Model file for the job. Use its own axes, mm. Face numbers are marked on the shaded views. Give positions to 0.01 mm unless a question says otherwise; leave off trailing zeros. Write each loop counter-clockwise with the first axis right and the second up, starting at its lowest first coordinate (ties: lowest second). Pieces come first, ordered by that corner, then holes. Notation, with made-up numbers: M 73,76.5 L 107,76.5 A24 cw 107,109.5 Z; hole C 81,-18 d9. An arc over 180 degrees is marked long. Answer as a JSON object with one key per item and string values. Group by question number.
```python
from build123d import *

# Parameters (mm, degrees)
CYLINDER002_R     = 1.5
CYLINDER002_DEPTH = 20
BOX033_W          = 12
BOX033_H          = 10
BOX033_DEPTH      = 12
FILLET011_R       = 4.5
FILLET012_R       = 4.6


with BuildPart() as cylinder:
    # Cylinder002 → Cylinder002 (new body)
    with BuildSketch(Plane(origin=(-103.2, 5, -48.3), x_dir=(1, 0, 0), z_dir=(0, 0, 1))):
        Circle(CYLINDER002_R)
    extrude(amount=CYLINDER002_DEPTH)


with BuildPart() as fillet012:
    # Box033 → Box033 (new body)
    with BuildSketch(Plane(origin=(-108.3, 0, -49.2), x_dir=(1, 0, 0), z_dir=(0, 0, 1))):
        with Locations((6, 5)):
            Rectangle(BOX033_W, BOX033_H)
    extrude(amount=BOX033_DEPTH)

    # Cut017: cut Cylinder
    add(cylinder.part, mode=Mode.SUBTRACT)

    # Fillet011
    fillet011_edges = [fillet012.edges().sort_by_distance(p)[0] for p in [
        (-108.3, 10, -43.2),
    ]]
    fillet(fillet011_edges, radius=FILLET011_R)

    # Fillet012
    fillet012_edges = [fillet012.edges().sort_by_distance(p)[0] for p in [
        (-108.3, 0, -43.2),
    ]]
    fillet(fillet012_edges, radius=FILLET012_R)


with BuildPart() as fillet012_1:
    # Fillet012 placement: moved
    add(fillet012.part.moved(Location((40.69, -41.14, 42.87))))


solid = fillet012_1.part
```
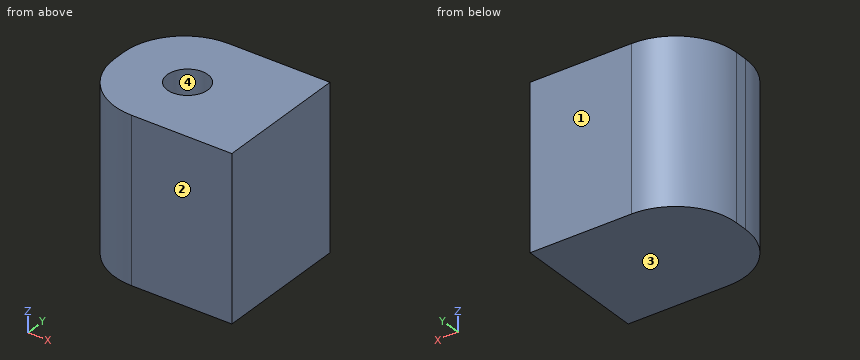
Q1. Two-plate mould, pull along Y, no slides. Class the marked faces 1, 2, 3 and 4: +Y half, -Y half, draft (parallel to the pull), parting line (faces both ways), or undercut.
Q2. Wall check: L1, parallel to X at y = -36.14, z = 2; L2, parallel to X at y = -36.5, z = -4.75; L3, parallel to X at y = -38, z = -1.25. Give the ranges that are in metal, low to high.
Q3. Drop flat-ended pins along their axis: P1, Ø2, axis at y = -33.5, z = 3, coming from the -X side; P2, Ø1, axis at x = -65, z = 1, coming from the +Y side. Give the stop position or say it passes through.
Q4. Slice it at B-B, the plane z = 4. Write the cut outline in (x, y).
Q5. Slice it at A-A, the plane x = -62.51. Write the cut outline in (y, z).
Q6. Slice it at C-C, the plane y = -36.14. Write the cut outline in (x, z).
Q7. Slice it at D-D, the plane y = -39. Write the cut outline in (x, z), then the cut area to 3 significant figures.
Solved:
{
 "1": {"face 1": "+Y half", "face 2": "-Y half", "face 3": "draft", "face 4": "undercut"},
 "2": {"L1": "x = -67.61 to -64.01, -61.01 to -55.61", "L2": "x = -67.61 to -63.97, -61.05 to -55.61", "L3": "x = -67.37 to -55.61"},
 "3": {"P1": "stops at x = -67.46", "P2": "stops at y = -31.36"},
 "4": {"outline": "M -67.61,-36.54 A4.6 ccw -63.01,-41.14 L -55.61,-41.14 L -55.61,-31.14 L -63.11,-31.14 A4.5 ccw -67.61,-35.64 Z; hole C -62.51,-36.14 d3"},
 "5": {"outline": "M -41.14,-6.33 L -31.14,-6.33 L -31.14,5.67 L -34.64,5.67 L -34.64,-5.43 L -37.64,-5.43 L -37.64,5.67 L -41.14,5.67 Z"},
 "6": {"outline": "M -67.61,-6.33 L -55.61,-6.33 L -55.61,5.67 L -61.01,5.67 L -61.01,-5.43 L -64.01,-5.43 L -64.01,5.67 L -67.61,5.67 Z"},
 "7": {"outline": "M -66.9,-6.33 L -55.61,-6.33 L -55.61,5.67 L -66.9,5.67 Z", "area": "135 mm²"}
}
